Drawing for the job (mm, zero at the part's lowest x, y, z). A direction names the side the tool comes from. Give positions to 0.01 mm unless a question says otherwise; leave off trailing zeros. Write each loop counter-clockwise with the first axis right and the second up, starting at its lowest first coordinate (ties: lowest second). Pieces come first, ordered by that corner, then holes. Notation, with made-up numbers: M 16.5,27 L 49.5,27 A3 ccw 49.5,32 Z; hole C 54.25,-21 d2. An arc over 180 degrees is marked long. Write item = value, one per line. Start each with the question number.
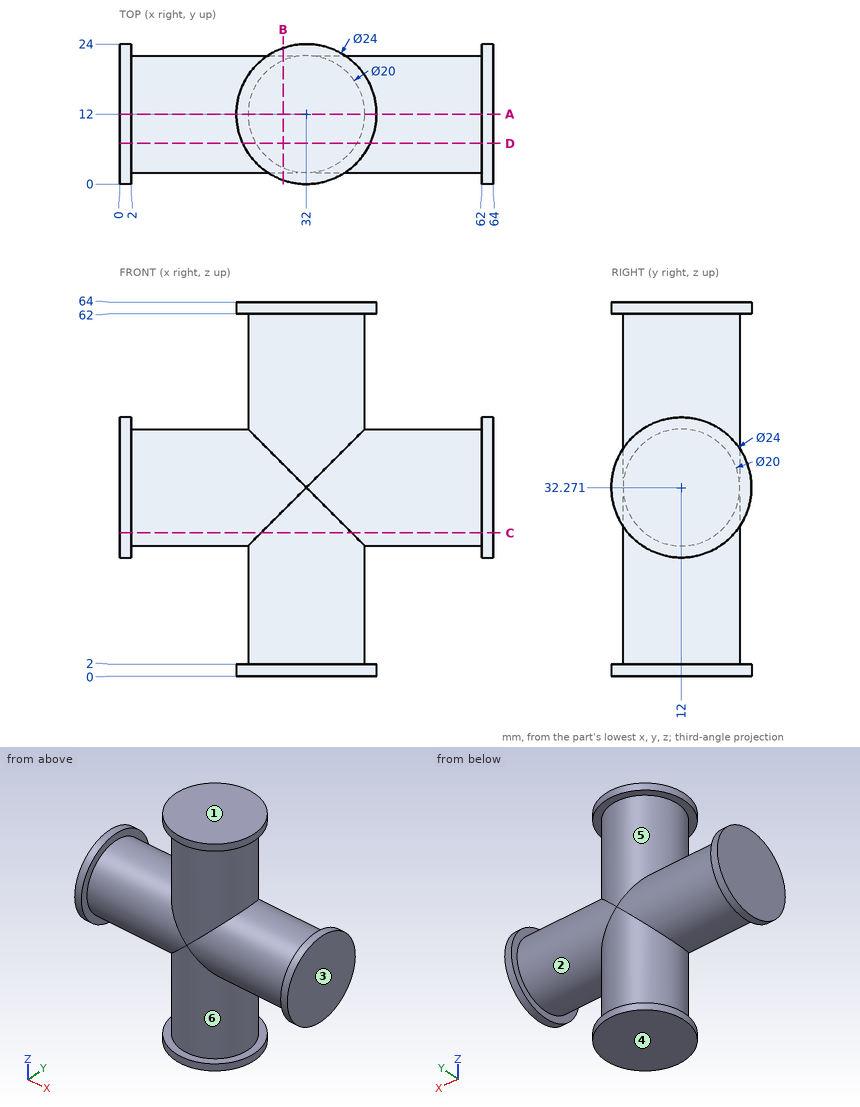
Q1. Slice it at C-C (z = 24.5). Give the cut face in (x, y).
Q2. Slice it at A-A (y = 12). Give the cut face in (x, z), and give its area (3 significant figures).
Q3. Slice it at B-B (x = 28). Give the cut face in (y, z) (1 decimal), and give its area (3 significant figures).
Q4. Drop flat-ended pins along their axis: P1, Ø7, axis at y = 17, z = 37, coming from the -X side; P2, Ø5, axis at x = 12.5, z = 29.5, coming from the +Y side; P3, Ø10, axis at x = 12.5, y = 7, coming from the -Z side; P4, Ø8, axis at y = 19.5, z = 51.5, coming from the +X side. Give the stop position or say it passes through.
Q5. Tool access for the marked faces 1 and 2: list every direction of +Z, -Z, +X, -X, +Y, -Y with a clear straight run to the whole face (end or side of a thin tool).
Q6. Two-plate mould, pull along Z, no slides. Class the marked faces 3, 4, 5 and 6: +Z half, -Z half, draft (parallel to the pull), parting line (faces both ways), or undercut.
Q7. Probe line 1 along X through (y, z) = (11.5, 43); line 2 along Y through (x, z) = (32, 31.5); line 3 along X through (y, z) = (12.25, 59.5). List the from-to ranges inside material, lowest first.
Q8. Slice it at D-D (y = 7). Give the cut face in (x, z), and give its area (3 significant figures).
Working result:
q1.outline = M 0,2.86 L 2,2.86 L 2,5.71 L 24.23,5.71 A10 ccw 39.77,5.71 L 62,5.71 L 62,2.86 L 64,2.86 L 64,21.14 L 62,21.14 L 62,18.29 L 39.77,18.29 A10 ccw 24.23,18.29 L 2,18.29 L 2,21.14 L 0,21.14 Z
q2.outline = M 0,20.27 L 2,20.27 L 2,22.27 L 22,22.27 L 22,2 L 20,2 L 20,0 L 44,0 L 44,2 L 42,2 L 42,22.27 L 62,22.27 L 62,20.27 L 64,20.27 L 64,44.27 L 62,44.27 L 62,42.27 L 42,42.27 L 42,62 L 44,62 L 44,64 L 20,64 L 20,62 L 22,62 L 22,42.27 L 2,42.27 L 2,44.27 L 0,44.27 Z
q2.area = 2,190 mm2
q3.outline = M 0.7,0 L 23.3,0 L 23.3,2 L 21.2,2 L 21.2,28.3 A10 ccw 21.2,36.3 L 21.2,62 L 23.3,62 L 23.3,64 L 0.7,64 L 0.7,62 L 2.8,62 L 2.8,36.3 A10 ccw 2.8,28.3 L 2.8,2 L 0.7,2 Z
q3.area = 1,200 mm2
q4.P1 = 0
q4.P2 = 22
q4.P3 = 22.27
q4.P4 = 41.37
q5.face_1 = +Z, +X, -X, +Y, -Y
q5.face_2 = none
q6.face_3 = draft
q6.face_4 = -Z half
q6.face_5 = undercut
q6.face_6 = undercut
q7.line_1 = 0 to 2, 22.01 to 41.99, 62 to 64
q7.line_2 = 2 to 22
q7.line_3 = 22 to 42
q8.outline = M 0,21.36 L 2,21.36 L 2,23.61 L 23.34,23.61 L 23.34,2 L 21.09,2 L 21.09,0 L 42.91,0 L 42.91,2 L 40.66,2 L 40.66,23.61 L 62,23.61 L 62,21.36 L 64,21.36 L 64,43.18 L 62,43.18 L 62,40.93 L 40.66,40.93 L 40.66,62 L 42.91,62 L 42.91,64 L 21.09,64 L 21.09,62 L 23.34,62 L 23.34,40.93 L 2,40.93 L 2,43.18 L 0,43.18 Z
q8.area = 1,950 mm2
